Read the model definition and answer for the solid it produces. Units are mm, in the model's axes. Coordinates: 2 decimals unless noted, no trailing zeros. Order: outer loops, then holes, each group sorted by start corner. A loop starts at its lowest first (then second) coordinate and runs counter-clockwise, first axis right, second up. Notation, with made-up numbers: (19.25, 18.5) -> (58.25, 18.5) arc R31 ccw to (58.25, 54.5) -> close; hole circle Ø11 at (71, 21). An arc over 180 degrees is marked (long way). Answer in a Markdown table with one row per item.
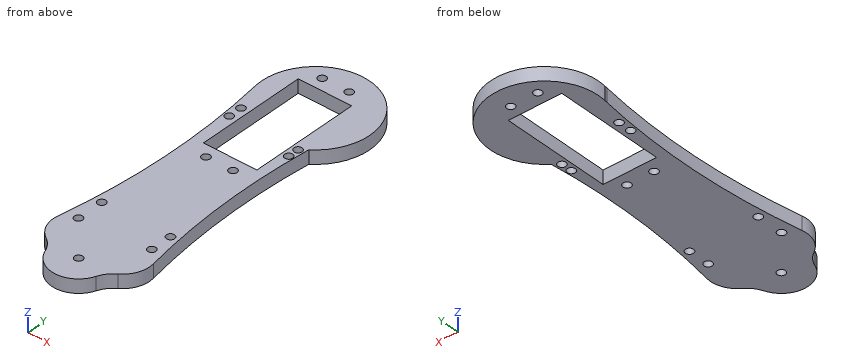
from build123d import *

# Parameters (mm, degrees)
RESSALTO_EXTRUS_O1_DEPTH = 5
FILETE3_R                = 10
FILETE4_R                = 10
ESBO_O2_R                = 1.5
CORTE_EXTRUS_O1_DEPTH    = 5
ESBO_O4_R                = 1.5
CORTE_EXTRUS_O3_DEPTH    = 10
ESBO_O5_W                = 19.8
ESBO_O5_H                = 40.6
CORTE_EXTRUS_O4_DEPTH    = 10
ESBO_O6_R                = 1.5
CORTE_EXTRUS_O5_DEPTH    = 10
ESBO_O7_R                = 1.5
CORTE_EXTRUS_O6_DEPTH    = 121.092170275


with BuildPart() as part:
    # Esboço1 → Ressalto-extrusão1 (new body)
    with BuildSketch(Plane.XY):
        with BuildLine():
            ThreePointArc((-10, 0), (0, -10), (10, 0))
            Line((10, 0), (20, 0))
            ThreePointArc((20, 0), (14.071698091, 40.495175194), (14.829943665, 81.414963086))
            ThreePointArc((14.829943665, 81.414963086), (11.193742071, 116.066691762), (-16.576524471, 95.024435265))
            Line((-16.576524471, 95.024435265), (-16.487894969, 94.437265709))
            Line((-16.487894969, 94.437265709), (-16.369382775, 93.652123615))
            ThreePointArc((-16.369382775, 93.652123615), (-13.756795166, 46.654405302), (-20, 0))
            Line((-20, 0), (-10, 0))
        make_face()
    extrude(amount=RESSALTO_EXTRUS_O1_DEPTH)

    # Filete3
    # the kernel refuses this fillet: 10 mm, written as the material it takes off along each edge
    with BuildSketch(Plane(origin=(20, 0, -29.463728433), x_dir=(-0.20232831186330175, 0.9793177493635794, 0), z_dir=(0, 0, 1))) as filete3_piece_1:
        with BuildLine():
            CenterArc((12.021201201, 9.997221658), FILETE3_R, 181.169168083, 87.480189)
            Line((2.023283119, 9.793177494), (1.823324757, 9.78909661))
            ThreePointArc((1.823324757, 9.78909661), (0.815778009, 4.937054409), (-0.19586355, 0.040465662))
            Line((-0.19586355, 0.040465662), (0.004714197, -0.199944433))
            ThreePointArc((0.004714197, -0.199944433), (5.892745687, -0.130541448), (11.780777177, -0.199944433))
            Line((11.780777177, -0.199944433), (11.785491373, 0))
        make_face()
    extrude(amount=63.927456867, mode=Mode.SUBTRACT)
    with BuildSketch(Plane(origin=(-20, 0, -29.463728433), x_dir=(1, 0, 0), z_dir=(0, 0, 1))) as filete3_piece_2:
        with BuildLine():
            CenterArc((12.222685959, 9.749854723), FILETE3_R, 169.67749742, 87.480189)
            Line((2.384538574, 11.541740887), (2.187775626, 11.57757861))
            ThreePointArc((2.187775626, 11.57757861), (1.06442773, 5.797282674), (-0.194855317, 0.045071116))
            Line((-0.194855317, 0.045071116), (0, -0.2))
            ThreePointArc((0, -0.2), (5, -0.2), (9.955546281, -0.194997094))
            Line((9.955546281, -0.194997094), (10, 0))
        make_face()
    extrude(amount=63.927456867, mode=Mode.SUBTRACT)

    # Filete4
    filete4_edges = [part.edges().sort_by_distance(p)[0] for p in [
        (10, 0, 2.5),
        (-10, 0, 2.5),
    ]]
    fillet(filete4_edges, radius=FILETE4_R)

    # Esboço2 → Corte-extrusão1 (cut)
    with BuildSketch(Plane.XY.offset(5)):
        Circle(ESBO_O2_R)
    extrude(amount=-CORTE_EXTRUS_O1_DEPTH, mode=Mode.SUBTRACT)

    # Esboço4 → Corte-extrusão3 (cut)
    with BuildSketch(Plane.XY.offset(5)):
        with Locations((-4.732435028, 109.78)):
            Circle(ESBO_O4_R)
        with Locations((5.267564972, 109.78)):
            Circle(ESBO_O4_R)
        with Locations((-4.732435028, 60)):
            Circle(ESBO_O4_R)
        with Locations((5.267564972, 60)):
            Circle(ESBO_O4_R)
    extrude(amount=-CORTE_EXTRUS_O3_DEPTH, mode=Mode.SUBTRACT)

    # Esboço5 → Corte-extrusão4 (cut)
    with BuildSketch(Plane.XY.offset(5)):
        with Locations((0.267564972, 84.89)):
            Rectangle(ESBO_O5_W, ESBO_O5_H)
    extrude(amount=-CORTE_EXTRUS_O4_DEPTH, mode=Mode.SUBTRACT)

    # Esboço6 → Corte-extrusão5 (cut)
    with BuildSketch(Plane(origin=(0, 0, 0), x_dir=(-1, 0, 0), z_dir=(0, 0, -1))):
        with Locations((12.6, 14.5)):
            Circle(ESBO_O6_R)
        with Locations((12.6, 24.5)):
            Circle(ESBO_O6_R)
        with Locations((12.6, 79.11)):
            Circle(ESBO_O6_R)
        with Locations((12.6, 84.11)):
            Circle(ESBO_O6_R)
    extrude(amount=-CORTE_EXTRUS_O5_DEPTH, mode=Mode.SUBTRACT)

    # Esboço7 → Corte-extrusão6 (cut, through all)
    with BuildSketch(Plane(origin=(0, 0, 0), x_dir=(-1, 0, 0), z_dir=(0, 0, -1))):
        with Locations((-12.77, 16.54)):
            Circle(ESBO_O7_R)
        with Locations((-12.77, 24.54)):
            Circle(ESBO_O7_R)
        with Locations((-12.57, 75.41)):
            Circle(ESBO_O7_R)
        with Locations((-12.57, 79.41)):
            Circle(ESBO_O7_R)
    extrude(amount=-CORTE_EXTRUS_O6_DEPTH, mode=Mode.SUBTRACT)


solid = part.part
Q1. The part is cut by section B-B (x = 0). Write down the section's boundary in (y, z).
Outcome:
| item | result |
|---|---|
| outline | (-10, 0) -> (-1.5, 0) -> (-1.5, 5) -> (-10, 5) -> close; (1.5, 0) -> (64.59, 0) -> (64.59, 5) -> (1.5, 5) -> close; (105.19, 0) -> (117.45, 0) -> (117.45, 5) -> (105.19, 5) -> close |
Q2. The part is cut by section D-D (y = 31.5). Write down the section's boundary in (x, z), then the cut area to 3 significant figures.
Outcome:
| item | result |
|---|---|
| outline | (-14.81, 0) -> (14.81, 0) -> (14.81, 5) -> (-14.81, 5) -> close |
| area | 148 mm² |
Q3. Given pin 1 (2.5 mm diameter, centred on x = 4.5, z = 1.5, fed in from -Y); pin 2 (3 mm diameter, centred on y = 91, z = 3.5, fed in from +X); pin 3 (1.5 mm diameter, centred on x = 1, z = 1.5, fed in from -Y), each flat-ended and moving along its own axis, determine where each tip first touches the part or whether it passes through.
Outcome:
| item | result |
|---|---|
| pin 1 | y = -9.46 |
| pin 2 | x = 22.55 |
| pin 3 | y = -10 |
Q4. The part is cut by section A-A (y = 84.11). Write down the section's boundary in (x, z).
Outcome:
| item | result |
|---|---|
| outline | (-15.12, 0) -> (-14.1, 0) -> (-14.1, 5) -> (-15.12, 5) -> close; (-11.1, 0) -> (-9.63, 0) -> (-9.63, 5) -> (-11.1, 5) -> close; (10.17, 0) -> (17.9, 0) -> (17.9, 5) -> (10.17, 5) -> close |
Q5. Consider line 1 (X direction, y = 95, z = 1.9); line 2 (X direction, y = 15.5, z = 3.55); line 3 (X direction, y = 94.5, z = 3.8). Determine where each line is inside the solid, lowest interval first.
Outcome:
| item | result |
|---|---|
| line 1 | -16.57 to -9.63, 10.17 to 23.06 |
| line 2 | -16.93 to -13.72, -11.48 to 11.69, 13.85 to 16.93 |
| line 3 | -16.5 to -9.63, 10.17 to 22.98 |
Q6. The part is cut by section C-C (z = 2.05). Give the number of separate pieces and of enclosed holes in the cut face, then the cut area to 3 significant figures.
Outcome:
| item | result |
|---|---|
| separate pieces | 1 |
| enclosed holes | 14 |
| area | 2,900 mm² |
